```python
from build123d import *

# Parameters (mm, degrees)
BOSS_EXTRUDE1_DEPTH = 19


with BuildPart() as part:
    # Sketch1 → Boss-Extrude1 (new body)
    with BuildSketch(Plane.XY):
        with BuildLine():
            Line((18, 65), (21.9, 65))
            ThreePointArc((21.9, 65), (24.021320344, 65.878679656), (24.9, 68))
            Line((24.9, 68), (24.9, 77))
            ThreePointArc((24.9, 77), (25.778679656, 79.121320344), (27.9, 80))
            Line((27.9, 80), (36.9, 80))
            ThreePointArc((36.9, 80), (39.021320344, 79.121320344), (39.9, 77))
            Line((39.9, 77), (39.9, 68))
            ThreePointArc((39.9, 68), (40.778679656, 65.878679656), (42.9, 65))
            Line((42.9, 65), (46.85, 65))
            ThreePointArc((46.85, 65), (48.971320344, 65.878679656), (49.85, 68))
            Line((49.85, 68), (49.85, 77))
            ThreePointArc((49.85, 77), (50.728679656, 79.121320344), (52.85, 80))
            Line((52.85, 80), (61.85, 80))
            ThreePointArc((61.85, 80), (63.971320344, 79.121320344), (64.85, 77))
            Line((64.85, 77), (64.85, 68))
            ThreePointArc((64.85, 68), (65.728679656, 65.878679656), (67.85, 65))
            Line((67.85, 65), (71.85, 65))
            ThreePointArc((71.85, 65), (73.971320344, 65.878679656), (74.85, 68))
            Line((74.85, 68), (74.85, 77))
            ThreePointArc((74.85, 77), (75.728679656, 79.121320344), (77.85, 80))
            Line((77.85, 80), (86.85, 80))
            ThreePointArc((86.85, 80), (88.971320344, 79.121320344), (89.85, 77))
            Line((89.85, 77), (89.85, 68))
            ThreePointArc((89.85, 68), (90.728679656, 65.878679656), (92.85, 65))
            Line((92.85, 65), (96.9, 65))
            ThreePointArc((96.9, 65), (99.021320344, 65.878679656), (99.9, 68))
            Line((99.9, 68), (99.9, 77))
            ThreePointArc((99.9, 77), (100.778679656, 79.121320344), (102.9, 80))
            Line((102.9, 80), (111.9, 80))
            ThreePointArc((111.9, 80), (114.021320344, 79.121320344), (114.9, 77))
            Line((114.9, 77), (114.9, 68))
            ThreePointArc((114.9, 68), (115.778679656, 65.878679656), (117.9, 65))
            Line((117.9, 65), (122, 65))
            ThreePointArc((122, 65), (124.121320344, 65.878679656), (125, 68))
            Line((125, 68), (125, 77))
            ThreePointArc((125, 77), (125.878679656, 79.121320344), (128, 80))
            Line((128, 80), (137, 80))
            ThreePointArc((137, 80), (139.121320344, 79.121320344), (140, 77))
            Line((140, 77), (140, 68))
            ThreePointArc((140, 68), (140.878679656, 65.878679656), (143, 65))
            Line((143, 65), (147.15, 65))
            ThreePointArc((147.15, 65), (149.271320344, 65.878679656), (150.15, 68))
            Line((150.15, 68), (150.15, 77))
            ThreePointArc((150.15, 77), (151.028679656, 79.121320344), (153.15, 80))
            Line((153.15, 80), (162.15, 80))
            ThreePointArc((162.15, 80), (164.271320344, 79.121320344), (165.15, 77))
            Line((165.15, 77), (165.15, 68))
            ThreePointArc((165.15, 68), (166.028679656, 65.878679656), (168.15, 65))
            Line((168.15, 65), (172.35, 65))
            ThreePointArc((172.35, 65), (174.471320344, 65.878679656), (175.35, 68))
            Line((175.35, 68), (175.35, 77))
            ThreePointArc((175.35, 77), (176.228679656, 79.121320344), (178.35, 80))
            Line((178.35, 80), (187.35, 80))
            ThreePointArc((187.35, 80), (189.471320344, 79.121320344), (190.35, 77))
            Line((190.35, 77), (190.35, 42))
            ThreePointArc((190.35, 42), (189.471320344, 39.878679656), (187.35, 39))
            Line((187.35, 39), (174.592640687, 39))
            ThreePointArc((174.592640687, 39), (170.35, 39), (170.35, 34.757359313))
            Line((170.35, 34.757359313), (170.35, 24.242640687))
            ThreePointArc((170.35, 24.242640687), (170.35, 20), (174.592640687, 20))
            Line((174.592640687, 20), (187.35, 20))
            ThreePointArc((187.35, 20), (189.471320344, 19.121320344), (190.35, 17))
            Line((190.35, 17), (190.35, 3))
            ThreePointArc((190.35, 3), (189.471320344, 0.878679656), (187.35, 0))
            Line((187.35, 0), (3, 0))
            ThreePointArc((3, 0), (0.878679656, 0.878679656), (0, 3))
            Line((0, 3), (0, 77))
            ThreePointArc((0, 77), (0.878679656, 79.121320344), (3, 80))
            Line((3, 80), (12, 80))
            ThreePointArc((12, 80), (14.121320344, 79.121320344), (15, 77))
            Line((15, 77), (15, 68))
            ThreePointArc((15, 68), (15.878679656, 65.878679656), (18, 65))
        make_face()
        with BuildLine():
            Line((31.694947257, 53.008010391), (35.694947257, 53.008010391))
            ThreePointArc((35.694947257, 53.008010391), (37.8162676, 52.129330734), (38.694947257, 50.008010391))
            Line((38.694947257, 50.008010391), (38.694947257, 41.008010391))
            ThreePointArc((38.694947257, 41.008010391), (39.573626913, 38.886690047), (41.694947257, 38.008010391))
            Line((41.694947257, 38.008010391), (54.694947257, 38.008010391))
            ThreePointArc((54.694947257, 38.008010391), (56.8162676, 38.886690047), (57.694947257, 41.008010391))
            Line((57.694947257, 41.008010391), (57.694947257, 50.008010391))
            ThreePointArc((57.694947257, 50.008010391), (58.573626913, 52.129330734), (60.694947257, 53.008010391))
            Line((60.694947257, 53.008010391), (64.694947257, 53.008010391))
            ThreePointArc((64.694947257, 53.008010391), (66.8162676, 52.129330734), (67.694947257, 50.008010391))
            Line((67.694947257, 50.008010391), (67.694947257, 41.008010391))
            Line((67.694947257, 41.008010391), (67.694947257, 29.736314532))
            ThreePointArc((67.694947257, 29.736314532), (66.8162676, 27.614994188), (64.694947257, 26.736314532))
            Line((64.694947257, 26.736314532), (56.194947257, 26.736314532))
            ThreePointArc((56.194947257, 26.736314532), (54.073626913, 25.857634875), (53.194947257, 23.736314532))
            Line((53.194947257, 23.736314532), (53.194947257, 14.736314532))
            ThreePointArc((53.194947257, 14.736314532), (52.3162676, 12.614994188), (50.194947257, 11.736314532))
            Line((50.194947257, 11.736314532), (46.194947257, 11.736314532))
            ThreePointArc((46.194947257, 11.736314532), (44.073626913, 12.614994188), (43.194947257, 14.736314532))
            Line((43.194947257, 14.736314532), (43.194947257, 23.736314532))
            ThreePointArc((43.194947257, 23.736314532), (42.3162676, 25.857634875), (40.194947257, 26.736314532))
            Line((40.194947257, 26.736314532), (31.694947257, 26.736314532))
            ThreePointArc((31.694947257, 26.736314532), (29.573626913, 27.614994188), (28.694947257, 29.736314532))
            Line((28.694947257, 29.736314532), (28.694947257, 41.008010391))
            Line((28.694947257, 41.008010391), (28.694947257, 50.008010391))
            ThreePointArc((28.694947257, 50.008010391), (29.573626913, 52.129330734), (31.694947257, 53.008010391))
        make_face(mode=Mode.SUBTRACT)
        with BuildLine():
            Line((90.694947257, 16.508010391), (90.694947257, 20.508010391))
            ThreePointArc((90.694947257, 20.508010391), (91.573626913, 22.629330734), (93.694947257, 23.508010391))
            Line((93.694947257, 23.508010391), (102.694947257, 23.508010391))
            ThreePointArc((102.694947257, 23.508010391), (104.8162676, 24.386690047), (105.694947257, 26.508010391))
            Line((105.694947257, 26.508010391), (105.694947257, 39.508010391))
            ThreePointArc((105.694947257, 39.508010391), (104.8162676, 41.629330734), (102.694947257, 42.508010391))
            Line((102.694947257, 42.508010391), (93.694947257, 42.508010391))
            ThreePointArc((93.694947257, 42.508010391), (91.573626913, 43.386690047), (90.694947257, 45.508010391))
            Line((90.694947257, 45.508010391), (90.694947257, 49.508010391))
            ThreePointArc((90.694947257, 49.508010391), (91.573626913, 51.629330734), (93.694947257, 52.508010391))
            Line((93.694947257, 52.508010391), (102.694947257, 52.508010391))
            Line((102.694947257, 52.508010391), (113.966643115, 52.508010391))
            ThreePointArc((113.966643115, 52.508010391), (116.087963459, 51.629330734), (116.966643115, 49.508010391))
            Line((116.966643115, 49.508010391), (116.966643115, 41.008010391))
            ThreePointArc((116.966643115, 41.008010391), (117.845322772, 38.886690047), (119.966643115, 38.008010391))
            Line((119.966643115, 38.008010391), (128.966643115, 38.008010391))
            ThreePointArc((128.966643115, 38.008010391), (131.087963459, 37.129330734), (131.966643115, 35.008010391))
            Line((131.966643115, 35.008010391), (131.966643115, 31.008010391))
            ThreePointArc((131.966643115, 31.008010391), (131.087963459, 28.886690047), (128.966643115, 28.008010391))
            Line((128.966643115, 28.008010391), (119.966643115, 28.008010391))
            ThreePointArc((119.966643115, 28.008010391), (117.845322772, 27.129330734), (116.966643115, 25.008010391))
            Line((116.966643115, 25.008010391), (116.966643115, 16.508010391))
            ThreePointArc((116.966643115, 16.508010391), (116.087963459, 14.386690047), (113.966643115, 13.508010391))
            Line((113.966643115, 13.508010391), (102.694947257, 13.508010391))
            Line((102.694947257, 13.508010391), (93.694947257, 13.508010391))
            ThreePointArc((93.694947257, 13.508010391), (91.573626913, 14.386690047), (90.694947257, 16.508010391))
        make_face(mode=Mode.SUBTRACT)
    extrude(amount=BOSS_EXTRUDE1_DEPTH)


solid = part.part
```
Geometry: final body of the model. Coordinates: model frame, mm. A direction names the side the tool comes from. Coordinates: 2 decimals unless noted, no trailing zeros. Use a Markdown table: item, result. Add a question column.
(1) Access query for faces 5 (the flat face through (49.85, 72, 9)), 6 (the flat face through (38.695, 46, 9)), 7 (the flat face through (132, 80, 9)). Directions: +Z, -Z, +X, -X, +Y, -Y. A direction counts if a zero-diameter tool reaches every point of the face in a straight line with its end or side. Return the directions, or none.
(2) Line query: line 1 along X through (y, z) = (48, 14.5); line 2 along X through (y, z) = (32, 17); line 3 along Y through (x, z) = (178, 1.5). Output: solid intervals per line, ascending.
(3) Pin query (flat end, axial travel): pin 1 Ø3.5 at (x, z) = (145, 8.5) entering from +Y. Return the tip coordinate at first contact, or that it passes through.
(4) Mould query, pull axis X, two halves, no side actions, for faces 1 (the flat face through (43.195, 19, 9)), 2 (the flat face through (97, 41, 0)), 3 (the flat face through (190.35, 10, 9)), 4 (the flat face through (34, 53.008, 9)). Classes: pulls with the +X half, pulls with the -X half, needs draft (parallel to the pull), parting line crosses it, or undercut.
(5) Section query A-A, the plane z = 8.5. State how many separate pieces and enclosed holes the cut face has, plus the area to 3 significant figures.
Answer:
| question | item | result |
|---|---|---|
| 1 | face 5 | +Z, -Z, +Y |
| 1 | face 6 | +Z, -Z |
| 1 | face 7 | +Z, -Z, +X, -X, +Y |
| 2 | line 1 | x = 0 to 28.69, 38.69 to 57.69, 67.69 to 90.69, 116.97 to 190.35 |
| 2 | line 2 | x = 0 to 28.69, 67.69 to 105.69, 131.97 to 170.35 |
| 2 | line 3 | y = 0 to 20, 39 to 79.98 |
| 3 | pin 1 | stops at y = 65 |
| 4 | face 1 | undercut |
| 4 | face 2 | needs draft |
| 4 | face 3 | pulls with the +X half |
| 4 | face 4 | undercut |
| 5 | separate pieces | 1 |
| 5 | enclosed holes | 2 |
| 5 | area | 12,000 mm^2 |
